from build123d import *

# Parameters (mm, degrees)
F0_W     = 63.5
F0_H     = 38.1
F0_R     = 2.4257
F0_R_2   = 2.0193
F1_DEPTH = 3.175
F2_W     = 31.75
F2_H     = 22.225
F3_DEPTH = 3.176


with BuildPart() as f1:
    # F0 (on Top) → F1 (new body)
    with BuildSketch(Plane.XY):
        Rectangle(F0_W, F0_H)
        with Locations((-25.4, -12.7)):
            Circle(F0_R, mode=Mode.SUBTRACT)
        with Locations((25.4, -12.7)):
            Circle(F0_R, mode=Mode.SUBTRACT)
        with Locations((-25.4, 0)):
            Circle(F0_R, mode=Mode.SUBTRACT)
        with Locations((-18, 12.7)):
            Circle(F0_R_2, mode=Mode.SUBTRACT)
        with Locations((25.4, 0)):
            Circle(F0_R, mode=Mode.SUBTRACT)
        with Locations((18, 12.7)):
            Circle(F0_R_2, mode=Mode.SUBTRACT)
    extrude(amount=F1_DEPTH)

    # F2 (on face) → F3 (cut, through all)
    with BuildSketch(Plane.XY.offset(3.175)):
        with Locations((0, -7.9375)):
            Rectangle(F2_W, F2_H)
    extrude(amount=-F3_DEPTH, mode=Mode.SUBTRACT)


solid = f1.part
Could you check a few things on this model? Use its own coordinates, in mm. A direction names the side the tool comes from. Round coordinates to 2 decimals unless told otherwise and drop trailing zeros. Order: outer loops, then holes, each group sorted by start corner. A loop starts at its lowest first (then second) coordinate and runs counter-clockwise, first axis right, second up.
(1) Please list where these lines run through material, in increasing order: line 1 along Y through (x, z) = (25.4, 2.05); line 2 along X through (y, z) = (-9.5, 2.6) (3 decimals); line 3 along X through (y, z) = (-1.5, 0.35) (3 decimals).
Response values:
line 1: y = -19.05 to -15.13, -10.27 to -2.43, 2.43 to 19.05
line 2: x = -31.75 to -15.875, 15.875 to 31.75
line 3: x = -31.75 to -27.306, -23.494 to -15.875, 15.875 to 23.494, 27.306 to 31.75
(2) Imagine slicing it at A-A (x = -18). Write out the boundary of the cut face in (y, z) (3 decimals), plus the area to 3 significant figures.
Response values:
outline: (-19.05, 0) - (10.681, 0) - (10.681, 3.175) - (-19.05, 3.175) - close; (14.719, 0) - (19.05, 0) - (19.05, 3.175) - (14.719, 3.175) - close
area: 108 mm2
(3) Imagine slicing it at C-C (z = 2.15). Write out the boundary of the cut face in (x, y) (3 decimals), plus the area to 3 significant figures.
Response values:
outline: (-31.75, -19.05) - (-15.875, -19.05) - (-15.875, 3.175) - (15.875, 3.175) - (15.875, -19.05) - (31.75, -19.05) - (31.75, 19.05) - (-31.75, 19.05) - close; hole circle Ø4.851 at (-25.4, -12.7); hole circle Ø4.851 at (-25.4, 0); hole circle Ø4.039 at (-18, 12.7); hole circle Ø4.039 at (18, 12.7); hole circle Ø4.851 at (25.4, -12.7); hole circle Ø4.851 at (25.4, 0)
area: 1,610 mm2
(4) Imagine slicing it at D-D (x = 25.4). Write out the boundary of the cut face in (y, z) (3 decimals).
Response values:
outline: (-19.05, 0) - (-15.126, 0) - (-15.126, 3.175) - (-19.05, 3.175) - close; (-10.274, 0) - (-2.426, 0) - (-2.426, 3.175) - (-10.274, 3.175) - close; (2.426, 0) - (19.05, 0) - (19.05, 3.175) - (2.426, 3.175) - close
(5) Which directions (+Z, -Z, +X, -X, +Y, -Y) give clear straight access to the entire face, cutting with the end or side of a thin tool? Please do faces 4 (the flat face through (-15.875, -8, 2)), 5 (the flat face through (-24, -19.05, 2)).
Response values:
face 4: +Z, -Z, -Y
face 5: +Z, -Z, +X, -X, -Y
(6) Imagine slicing it at B-B (y = 12.7). Write out the boundary of the cut face in (x, z) (3 decimals), plus the area to 3 significant figures.
Response values:
outline: (-31.75, 0) - (-20.019, 0) - (-20.019, 3.175) - (-31.75, 3.175) - close; (-15.981, 0) - (15.981, 0) - (15.981, 3.175) - (-15.981, 3.175) - close; (20.019, 0) - (31.75, 0) - (31.75, 3.175) - (20.019, 3.175) - close
area: 176 mm2
(7) I'm going to push a flat-ended pin straight in: pin 1 (3 mm diameter, centred on x = -25.4, y = -12.7, fed in from -Z). Where does the tip first touch, or does it pass through?
Response values:
pin 1: passes through
(8) If we mould it in two halves opening along Y, with no side actions, what happens to faces 1 (the flat face through (0, 19.05, 2)), 2 (the flat face through (-31.75, 0, 2)), 3 (the cylindrical face through (22.977, 0.107, 1.565))? For each: released by +Y, released by -Y, zero draft, split by the parting line, or undercut.
Response values:
face 1: released by +Y
face 2: zero draft
face 3: undercut
